Verification items for the finished model (mm, model axes). Face numbers are marked on the shaded views. A direction names the side the tool comes from. Coordinates: 2 decimals unless noted, no trailing zeros. Write each loop counter-clockwise with the first axis right and the second up, starting at its lowest first coordinate (ties: lowest second). Pieces come first, ordered by that corner, then holes. Notation, with made-up numbers: (45.5, 8) - (53.5, 8) arc R29 ccw to (53.5, 36) - close; hole circle Ø1 at (38.25, -35.75). An arc over 180 degrees is marked (long way). Use one line per item in the form item = value. Start each with the question number.
(1) Sectioned sample at B-B (y = 25.5). Record the cut outline in (x, z), and give its area (3 significant figures).
(2) Sectioned sample at C-C (y = 14). Record the cut outline in (x, z).
(3) Sectioned sample at D-D (y = 48). Record the cut outline in (x, z).
(4) Sectioned sample at A-A (x = 25.4). Record the cut outline in (y, z).
(5) Tool access check on the marked faces 5, 6 and 7. Record the directions out of +Z, -Z, +X, -X, +Y, -Y that give a thin tool (end or side, any length) a straight path to the whole face; none if there is none.
(6) Mould release check, pull along Y, two halves, no side actions. Record for the marked faces 1, 2, 3 and 4: released by +Y, released by -Y, zero draft, split by the parting line, or undercut.
(7) Gauge pin test, flat ends, axial feed: pin 1 Ø1.5 at (y, z) = (28.5, 53.5) entering from +X; pin 2 Ø5 at (y, z) = (7.5, 13) entering from -X; pin 3 Ø4 at (x, y) = (104, 21) entering from +Z. Record the tip position at first contact, or that the pin passes through.
(8) Material ranges on line 1 (X direction, y = 25.4, z = 2); line 2 (Y direction, x = 63.5, z = 20) (3 decimals); line 3 (X direction, y = 14, z = 6.5), recorded low to high. Write a range as [from, to].
Autodesk Inventor part; units mm, degrees
ref_plane "YZ Plane" through (0, 0, 0) normal (1, 0, 0) x (0, 1, 0)
ref_plane "XZ Plane" through (0, 0, 0) normal (0, 1, 0) x (-1, 0, 0)
ref_plane "XY Plane" through (0, 0, 0) normal (0, 0, 1) x (1, 0, 0)
sketch "Sketch1" plane through (0, 0, 0) normal (0, 0, 1) x (1, 0, 0)
  line L0 (0, 0) -> (152.4, 0)
  line L1 (152.4, 0) -> (152.4, 50.8)
  line L2 (152.4, 50.8) -> (0, 50.8)
  line L3 (0, 50.8) -> (0, 0)
  dimension "d0" = 50.8
  dimension "d1" = 152.4
extrude "Extrusion1" add sketch "Sketch1" along normal blind 6.35
sketch "Sketch2" plane through (0, 0, 6.35) normal (0, 0, 1) x (1, 0, 0)
  line L0 (0, 0) -> (0, 50.8)
  line L1 (152.4, 50.8) -> (152.4, 0)
  point P0 (25.4, 25.4)
  point P1 (127, 25.4)
  point P2 (0, 25.4)
  dimension "d4" = 25.4
  dimension "d5" = 25.4
hole "Hole1" at (25.4, 25.4, 6.35) at (127, 25.4, 6.35) direction (0, 0, -1) diameter 7.62 end through all
sketch "Sketch3" plane through (0, 50.8, 0) normal (0, 1, 0) x (1, 0, 0)
  line L0 (0, -6.35) -> (152.4, -6.35)
  line L1 (0, 0) -> (0, -6.35)
  line L2 (101.8247, -6.35) -> (106.5326, -56.3502)
  line L3 (106.5326, -56.3502) -> (55.9563, -61.1124)
  line L4 (55.9563, -61.1124) -> (50.8, -6.35)
  dimension "d13" = 50.8
  dimension "d14" = 50.8
  dimension "d15" = 54.7624
  dimension "d16" = 5.379
extrude "Extrusion2" add sketch "Sketch3" against normal up to surface (50.8 mm away)
sketch "Sketch4" plane through (106.5326, 0, 56.3502) normal (0.0937434, 0, 0.9955964) x (0.9955964, 0, -0.0937434)
  line L0 (-50.8, 50.8) -> (0, 50.8)
  line L1 (-50.8, 50.8) -> (-50.8, 0)
  line L2 (-43.18, 46.355) -> (-7.62, 46.355)
  line L3 (-4.445, 43.18) -> (-4.445, 7.62)
  line L4 (-7.62, 4.445) -> (-43.18, 4.445)
  line L5 (-46.355, 7.62) -> (-46.355, 43.18)
  arc A0 (-43.18, 46.355) -> (-46.355, 43.18) centre (-43.18, 43.18) ccw
  arc A1 (-46.355, 7.62) -> (-43.18, 4.445) centre (-43.18, 7.62) ccw
  arc A2 (-7.62, 4.445) -> (-4.445, 7.62) centre (-7.62, 7.62) ccw
  arc A3 (-4.445, 43.18) -> (-7.62, 46.355) centre (-7.62, 43.18) ccw
  point P0 (-100.781, 0)
  point P1 (-25.4, 46.355)
  point P2 (-25.4, 50.8)
  point P3 (-46.355, 25.4)
  point P4 (-50.8, 25.4)
  dimension "d19" = 3.175
  dimension "d20" = 4.445
  dimension "d21" = 4.445
extrude "Extrusion3" cut sketch "Sketch4" against normal up to surface surface through (76.2, 25.4, 6.35) normal (0, 0, 1)
fillet "Fillet1" radius 6.35 4 edges at (53.3782, 50.8, 33.7312) (53.3782, 0, 33.7312) (104.1787, 50.8, 31.3501) (104.1787, 0, 31.3501)
hole "Hole2" at (78.8634, 50.8, 33.4432) direction (0, -1, 0) diameter 7.62 end through all
properties part number "short frame bracket" material "Steel"
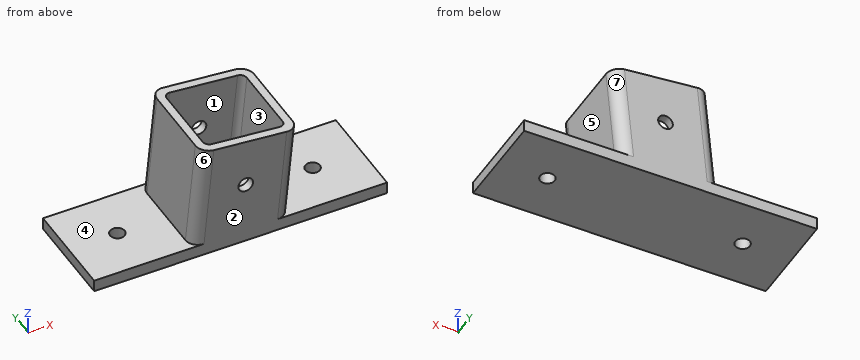
Answers below:
q1.outline = (0, 0) - (21.59, 0) - (21.59, 6.35) - (0, 6.35) - close; (29.21, 0) - (123.19, 0) - (123.19, 6.35) - (101.82, 6.35) - (106.53, 56.35) - (102.11, 56.77) - (97.36, 6.35) - (55.26, 6.35) - (60.38, 60.7) - (55.96, 61.11) - (50.8, 6.35) - (29.21, 6.35) - close; (130.81, 0) - (152.4, 0) - (152.4, 6.35) - (130.81, 6.35) - close
q1.area = 1,340 mm2
q2.outline = (0, 0) - (152.4, 0) - (152.4, 6.35) - (101.82, 6.35) - (106.53, 56.35) - (102.11, 56.77) - (97.36, 6.35) - (55.26, 6.35) - (60.38, 60.7) - (55.96, 61.11) - (50.8, 6.35) - (0, 6.35) - close
q3.outline = (0, 0) - (152.4, 0) - (152.4, 6.35) - (100.73, 6.35) - (105.45, 56.45) - (57.04, 61.01) - (51.89, 6.35) - (0, 6.35) - close; hole circle Ø7.62 at (78.86, 33.44)
q4.outline = (0, 0) - (21.59, 0) - (21.59, 6.35) - (0, 6.35) - close; (29.21, 0) - (50.8, 0) - (50.8, 6.35) - (29.21, 6.35) - close
q5.face_5 = +X, +Y, -Y
q5.face_6 = +Z, -X, -Y
q5.face_7 = +X, +Y
q6.face_1 = undercut
q6.face_2 = released by -Y
q6.face_3 = undercut
q6.face_4 = zero draft
q7.pin_1 = 106.33
q7.pin_2 = 51.19
q7.pin_3 = 56.77
q8.line_1 = [0, 21.59], [29.21, 123.19], [130.81, 152.4]
q8.line_2 = [0, 4.445], [46.355, 50.8]
q8.line_3 = [50.81, 55.28], [97.37, 101.84]
